```python
from build123d import *

# Parameters (mm, degrees)
SKETCH1_W           = 20
SKETCH1_H           = 25
SKETCH1_R           = 0.75
SKETCH1_R_2         = 1
BOSS_EXTRUDE1_DEPTH = 3


with BuildPart() as part:
    # Sketch1 → Boss-Extrude1 (new body)
    with BuildSketch(Plane.XY):
        with Locations((10, -12.5)):
            Rectangle(SKETCH1_W, SKETCH1_H)
        with Locations((10, -17)):
            Circle(SKETCH1_R, mode=Mode.SUBTRACT)
        with Locations((3, -10)):
            Circle(SKETCH1_R, mode=Mode.SUBTRACT)
        with BuildLine():
            ThreePointArc((10, -7), (12.121320344, -7.878679656), (13, -10))
            ThreePointArc((13, -10), (12.121320344, -12.121320344), (10, -13))
            ThreePointArc((10, -13), (7.878679656, -12.121320344), (7, -10))
            ThreePointArc((7, -10), (7.878679656, -7.878679656), (10, -7))
        make_face(mode=Mode.SUBTRACT)
        with Locations((10, -3)):
            Circle(SKETCH1_R, mode=Mode.SUBTRACT)
        with Locations((17, -10)):
            Circle(SKETCH1_R, mode=Mode.SUBTRACT)
        with Locations((4.5, -22.5)):
            Circle(SKETCH1_R_2, mode=Mode.SUBTRACT)
        with Locations((15.5, -22.5)):
            Circle(SKETCH1_R_2, mode=Mode.SUBTRACT)
    extrude(amount=BOSS_EXTRUDE1_DEPTH)


solid = part.part
```
CAD build for the part. Positions are in the model's coordinates, mm. Coordinates: 2 decimals unless noted, no trailing zeros. Loops run counter-clockwise (first coordinate to the right, second up) from the corner with the lowest first, then second, coordinate; pieces in that order, holes last. Notation, with made-up numbers: (-14.5, 23) - (22.5, 23) arc R26 ccw to (22.5, 61) - close; hole circle Ø7 at (-26, 51.5). An arc over 180 degrees is marked (long way). Use CSV: the item, a comma, the result in double quotes. Start each with the question number.
Q1. Probe probe 1 along Y at (x, z) = (3, 1.55); probe 2 along Y at (x, z) = (4.5, 2.1); probe 3 along X at (y, z) = (-8, 0.35). List the from-to ranges inside material, lowest first. Write a range as from..to.
Q2. Cut at B-B, the plane x = 17. List the corners of the cut face in (y, z).
Q3. Cut at A-A, the plane y = -22.5. List the corners of the cut face in (x, z).
Q4. Cut at D-D, the plane y = -17. List the corners of the cut face in (x, z).
Q5. Cut at C-C, the plane z = 1.5. List the corners of the cut face in (x, y).
Q6. Two-plate mould, pull along Y, no slides. Class faces 1 (the flat face through (10, -25, 1)), 2 (the flat face through (7.6, -12.3, 3)), 3 (the cylindrical face through (9.25, -2.97, 1.48)): +Y half, -Y half, draft (parallel to the pull), parting line (faces both ways), or undercut.
Here are the results:
1,probe 1,"-25..-10.75, -9.25..0"
1,probe 2,"-25..-23.5, -21.5..0"
1,probe 3,"0..7.76, 12.24..20"
2,outline,"(-25, 0) - (-10.75, 0) - (-10.75, 3) - (-25, 3) - close; (-9.25, 0) - (0, 0) - (0, 3) - (-9.25, 3) - close"
3,outline,"(0, 0) - (3.5, 0) - (3.5, 3) - (0, 3) - close; (5.5, 0) - (14.5, 0) - (14.5, 3) - (5.5, 3) - close; (16.5, 0) - (20, 0) - (20, 3) - (16.5, 3) - close"
4,outline,"(0, 0) - (9.25, 0) - (9.25, 3) - (0, 3) - close; (10.75, 0) - (20, 0) - (20, 3) - (10.75, 3) - close"
5,outline,"(0, -25) - (20, -25) - (20, 0) - (0, 0) - close; hole circle Ø1.5 at (3, -10); hole circle Ø2 at (4.5, -22.5); hole circle Ø6 at (10, -10); hole circle Ø1.5 at (10, -17); hole circle Ø1.5 at (10, -3); hole circle Ø2 at (15.5, -22.5); hole circle Ø1.5 at (17, -10)"
6,face 1,"-Y half"
6,face 2,"draft"
6,face 3,"undercut"
